```python
from build123d import *

# Parameters (mm, degrees)
SKETCH1_R                = 13
SKETCH1_R_2              = 7
BOSS_EXTRUDE2_DEPTH      = 10
SKETCH2_R                = 10
BOSS_EXTRUDE3_DEPTH      = 28
SKETCH3_R                = 10
SKETCH3_R_2              = 13
SKETCH3_R_3              = 7
BOSS_EXTRUDE4_DEPTH      = 10
SKETCH4_R                = 10
BOSS_EXTRUDE5_DEPTH      = 10
FILLET1_R                = 10
CUT_EXTRUDE1_DEPTH       = 17
BOSS_EXTRUDE6_DEPTH      = 28
BOSS_EXTRUDE6_DEPTH_BACK = 5
SKETCH6_R                = 5
FILLET2_R                = 10
SKETCH7_W                = 10
SKETCH7_H                = 10
BOSS_EXTRUDE7_DEPTH      = 10
BOSS_EXTRUDE8_DEPTH      = 9
BOSS_EXTRUDE8_DEPTH_BACK = 18
SKETCH8_R                = 5


with BuildPart() as part:
    # Sketch1 → Boss-Extrude2 (new body)
    # profile 1 of 2: a face of its own
    with BuildSketch(Plane(origin=(0, 0, 0), x_dir=(1, 0, 0), z_dir=(0, 1, 0))):
        with BuildLine():
            ThreePointArc((29.247640438, 60), (16.247640438, 47), (3.247640438, 60))
            Line((3.247640438, 60), (-5.462946679, 0))
            Line((-5.462946679, 0), (52.203983694, 0))
            Line((52.203983694, 0), (29.247640438, 60))
        make_face()
    # profile 2 of 2: a face of its own
    with BuildSketch(Plane(origin=(0, 0, 0), x_dir=(1, 0, 0), z_dir=(0, 1, 0))):
        with Locations((16.247640438, 60)):
            Circle(SKETCH1_R)
        with Locations(Location((16.247640438, 60, 0), (0, 0, 270))):
            Circle(SKETCH1_R_2, mode=Mode.SUBTRACT)
    extrude(amount=BOSS_EXTRUDE2_DEPTH)

    # Sketch2 → Boss-Extrude3 (add)
    with BuildSketch(Plane.XZ):
        with Locations(Location((16.05250876, -30, 0), (0, 0, 90))):
            Circle(SKETCH2_R)
    extrude(amount=BOSS_EXTRUDE3_DEPTH)



with BuildPart() as body_2:
    # Sketch3 → Boss-Extrude4 (new body)
    # profile 1 of 2: a face of its own
    with BuildSketch(Plane.XZ.offset(28)):
        with BuildLine():
            Line((-5.462946679, 0), (3.247640438, -60))
            ThreePointArc((3.247640438, -60), (16.247640438, -47), (29.247640438, -60))
            Line((29.247640438, -60), (52.203983694, 0))
            Line((52.203983694, 0), (-5.462946679, 0))
        make_face()
        with Locations(Location((16.05250876, -30, 0), (0, 0, 90))):
            Circle(SKETCH3_R, mode=Mode.SUBTRACT)
    # profile 2 of 2: a face of its own
    with BuildSketch(Plane.XZ.offset(28)):
        with Locations((16.247640438, -60)):
            Circle(SKETCH3_R_2)
        with Locations(Location((16.247640438, -60, 0), (0, 0, 90))):
            Circle(SKETCH3_R_3, mode=Mode.SUBTRACT)
    extrude(amount=BOSS_EXTRUDE4_DEPTH)


with BuildPart() as part_1:
    add(part.part)

    add(body_2.part)  # Boss-Extrude5 merges body 2
    # Sketch4 → Boss-Extrude5 (add)
    with BuildSketch(Plane.XZ.offset(28)):
        with Locations(Location((16.05250876, -30, 0), (0, 0, 90))):
            Circle(SKETCH4_R)
    extrude(amount=BOSS_EXTRUDE5_DEPTH)

    # Fillet1
    fillet1_edges = [part_1.edges().sort_by_distance(p)[0] for p in [
        (-5.462946679, -33, 0),
        (52.203983694, -33, 0),
    ]]
    fillet(fillet1_edges, radius=FILLET1_R)

    # Sketch5 → Cut-Extrude1 (cut)
    with BuildSketch(Plane.XY):
        Polygon((27.537053321, 10), (4.537053321, 10), (4.537053321, 5), (4.537053321, 0), (27.537053321, 0), align=None)
    extrude(amount=-CUT_EXTRUDE1_DEPTH, mode=Mode.SUBTRACT)

    # Sketch6 → Boss-Extrude6 (add, two sides: drawn at the far end of the back side and taken through both)
    with BuildSketch(Plane.ZY.offset(-27.537053321).offset(-BOSS_EXTRUDE6_DEPTH_BACK)):
        with Locations(Location((0, 5, 0), (0, 0, 90))):
            Circle(SKETCH6_R)
    extrude(amount=BOSS_EXTRUDE6_DEPTH + BOSS_EXTRUDE6_DEPTH_BACK)

    # Fillet2
    # the kernel refuses this fillet: 10 mm, written as the material it takes off along each edge
    with BuildSketch(Plane(origin=(52.203983694, -36.33251049, 0), x_dir=(-0.3573434345280911, 0, -0.9339730562493053), z_dir=(0, 1, 0))) as fillet2_piece_1:
        with BuildLine():
            CenterArc((FILLET2_R * 1.45330041958, FILLET2_R), FILLET2_R, 159.0628634, 110.9371366)
            Line((FILLET2_R * 0.519327363336, FILLET2_R * 1.35734343453), (FILLET2_R * 0.500647902211, FILLET2_R * 1.36449030322))
            Line((FILLET2_R * 0.500647902211, FILLET2_R * 1.36449030322), (-FILLET2_R * 0.0290660083917, -FILLET2_R * 0.02))
            Line((-FILLET2_R * 0.0290660083917, -FILLET2_R * 0.02), (FILLET2_R * 1.45330041958, -FILLET2_R * 0.02))
            Line((FILLET2_R * 1.45330041958, -FILLET2_R * 0.02), (FILLET2_R * 1.45330041958, 0))
        make_face()
    extrude(amount=82.665020979, mode=Mode.SUBTRACT)
    with BuildSketch(Plane(origin=(-5.462946679, -23.371123881, 0), x_dir=(1, 0, 0), z_dir=(0, 1, 0))) as fillet2_piece_2:
        with BuildLine():
            CenterArc((11.239350904, 7.814761692), FILLET2_R, 171.739711253, 59.656220213)
            Line((1.343094868, 9.251465031), (1.145169748, 9.280199097))
            Line((1.145169748, 9.280199097), (-0.197925121, 0.028734067))
            Line((-0.197925121, 0.028734067), (0, -0.2))
            ThreePointArc((0, -0.2), (2.5, -0.2), (4.875212982, -0.156295234))
            Line((4.875212982, -0.156295234), (5, 0))
        make_face()
    extrude(amount=56.742247763, mode=Mode.SUBTRACT)

    # Sketch7 → Boss-Extrude7 (add)
    with BuildSketch(Plane(origin=(0, -38, 0), x_dir=(-1, 0, 0), z_dir=(0, -1, 0))):
        with Locations((-16.093649369, 10.399188766)):
            Rectangle(SKETCH7_W, SKETCH7_H)
    extrude(amount=BOSS_EXTRUDE7_DEPTH)

    # Sketch8 → Boss-Extrude8 (add, two sides: drawn at the far end of the back side and taken through both)
    with BuildSketch(Plane(origin=(21.093649369, 0, 0), x_dir=(0, 0, -1), z_dir=(1, 0, 0)).offset(-BOSS_EXTRUDE8_DEPTH_BACK)):
        with Locations((10.399188766, -48)):
            Circle(SKETCH8_R)
    extrude(amount=BOSS_EXTRUDE8_DEPTH + BOSS_EXTRUDE8_DEPTH_BACK)


solid = part_1.part
```
The model under review builds one solid part; all positions refer to its coordinate system, in mm. A direction names the side the tool comes from. Coordinates: 2 decimals unless noted, no trailing zeros. Order: outer loops, then holes, each group sorted by start corner. A loop starts at its lowest first (then second) coordinate and runs counter-clockwise, first axis right, second up. Notation, with made-up numbers: M 29.5,32 L 36.5,32 A32 ccw 36.5,71 Z; hole C 10.25,9.5 d7. An arc over 180 degrees is marked long. One line per question, with ' | ' between items.
(1) Add section A-A, the plane x = 1. Write out the cut boundary in (y, z), then the cut area to 3 significant figures.
Geometry results:
outline: M -38,-44.52 L -28,-44.52 L -28,-1.39 L -38,-1.39 Z; M 0,-44.52 L 10,-44.52 L 10,0 A5 ccw 0,0 Z | area: 916 mm²
(2) For probe 1 along X at (y, z) = (-31.75, -60); probe 2 along Y at (x, z) = (31.5, -22.5); probe 3 along Z at (x, y) = (18.5, 5.5), list the stretches that pass through material, from the lowest coordinate up. Write a range as from..to.
Geometry results:
probe 1: x = 3.25..9.25, 23.25..29.25 | probe 2: y = -38..-28, 0..10 | probe 3: z = -72.8..-66.63, -53.37..-17, -4.97..4.97
(3) The part is to be moulded in two halves that separate along X. For faces 1 (the face through (25.815, -13.804, -32.168)), 2 (the face through (10.037, 4.93, -56.77)), 3 (the face through (-3.55, 4.93, -4.21)), say which applies: +X half, -X half, draft (parallel to the pull), parting line (faces both ways), or undercut.
Geometry results:
face 1: parting line | face 2: undercut | face 3: -X half
(4) Insertion check: pin 1 (4 mm diameter, centred on x = 3.5, y = -28.5, fed in from +Z); pin 2 (2.5 mm diameter, centred on y = 3, z = 3.5, fed in from -X); pin 3 (8 mm diameter, centred on y = -43, z = -8, fed in from +X); pin 4 (8 mm diameter, centred on y = 5, z = -12, fed in from +X). Each pin has a flat end and moves straight along its axis. Give the tip position at first contact, or say it passes through.
Geometry results:
pin 1: stops at z = -0.02 | pin 2: stops at x = -0.46 | pin 3: stops at x = 30.09 | pin 4: stops at x = 47.67
(5) Add section C-C, the plane y = -36. Write out the cut boundary in (x, z), then the cut area to 3 significant figures.
Geometry results:
outline: M -3.8,-11.44 L 3.25,-60 A13 ccw 29.25,-60 L 47.01,-13.57 A10 ccw 37.67,0 L 6.09,0 A10 ccw Z; hole C 16.25,-60 d14 | area: 2,540 mm²
(6) Add section B-B, the plane x = 20. Write out the cut boundary in (y, z).
Geometry results:
outline: M -48,-15.4 L -38,-15.4 L -38,-54.09 L -28,-54.09 L -28,-39.19 L 0,-39.19 L 0,-54.09 L 10,-54.09 L 10,-17 L 0,-17 L 0,-20.81 L -28,-20.81 L -28,0 L -38,0 L -38,-5.4 L -48,-5.4 A5 ccw Z; M -38,-72.45 L -28,-72.45 L -28,-65.91 L -38,-65.91 Z; M 0,-72.45 L 10,-72.45 L 10,-65.91 L 0,-65.91 Z; C 5,0 d10
(7) Machinability: for faces 4 (the face through (16, 5, -17)), 5 (the face through (-0.327, -32.93, -35.378)), 6 (the face through (32.537, 5, 2)), 7 (the face through (30.094, -48, -10)), 8 (the face through (15.962, -32.93, -72.997)), which of the approach directions +Z, -Z, +X, -X, +Y, -Y give a long, thin tool a straight path to every point of the face, cutting with its end or side? Answer none if there is none.
Geometry results:
face 4: +Y | face 5: -Z, -X, +Y, -Y | face 6: +Z, +X, +Y, -Y | face 7: +Z, -Z, +X, -Y | face 8: -Z, +Y, -Y
(8) Add section D-D, the plane z = -64.5. Write out the cut boundary in (x, y).
Geometry results:
outline: M 4.05,-38 L 10.89,-38 L 10.89,-28 L 4.05,-28 Z; M 4.05,0 L 10.89,0 L 10.89,10 L 4.05,10 Z; M 21.61,-38 L 28.44,-38 L 28.44,-28 L 21.61,-28 Z; M 21.61,0 L 28.44,0 L 28.44,10 L 21.61,10 Z
